```python
from build123d import *

# Parameters (mm, degrees)
EXTRUDE1_DEPTH     = 7.595616
EXTRUDE2_DEPTH     = 3.000375
CIRPATTERN1_COUNT  = 2
CIRPATTERN1_ANGLE  = 90
SKETCH4_R          = 5.969
CUT_EXTRUDE1_DEPTH = 39.496492
SKETCH7_R          = 1.8161
CUT_EXTRUDE2_DEPTH = 70.535078783


with BuildPart() as part:
    # Sketch1 → Revolve1 (revolve)
    with BuildSketch(Plane.XY, mode=Mode.PRIVATE) as revolve1_sk:
        Polygon((34.0487, 5.969), (34.0487, 7.1628), (32.5165085, 7.1628), (21.791168, 9.0424), (21.791168, 7.23392), (8.852662, 7.23392), (8.852662, 9.94664), (5.447792, 9.94664), (5.447792, 7.957312), (-5.447792, 7.957312), (-5.447792, 9.94664), (-8.852662, 9.94664), (-8.852662, 2.8575), (-25.6667, 2.8575), (-25.6667, 3.81), (-33.00095, 2.270125), (-34.0487, 2.270125), (-34.0487, 1.8161), (-5.447792, 1.8161), (-5.447792, 5.969), align=None)
    revolve(revolve1_sk.sketch.rotate(Axis((0, 0, 0), (1, 0, 0)), 90), axis=Axis((0, 0, 0), (1, 0, 0)))

    # Sketch2 → Revolve2 (revolve)
    with BuildSketch(Plane.XY, mode=Mode.PRIVATE) as revolve2_sk:
        with BuildLine():
            Line((10.661142, 7.23392), (8.852662, 7.23392))
            Line((8.852662, 7.23392), (8.852662, 9.0424))
            ThreePointArc((8.852662, 9.0424), (9.382353528, 7.763611528), (10.661142, 7.23392))
        make_face()
        with BuildLine():
            Line((5.447792, 9.94664), (5.447792, 7.957312))
            Line((5.447792, 7.957312), (3.458464, 7.957312))
            ThreePointArc((3.458464, 7.957312), (4.865131319, 8.539972681), (5.447792, 9.94664))
        make_face()
        with BuildLine():
            Line((-5.447792, 9.94664), (-5.447792, 7.957312))
            Line((-5.447792, 7.957312), (-3.458464, 7.957312))
            ThreePointArc((-3.458464, 7.957312), (-4.865131319, 8.539972681), (-5.447792, 9.94664))
        make_face()
        with BuildLine():
            Line((-12.397232, 2.8575), (-8.852662, 2.8575))
            Line((-8.852662, 2.8575), (-8.852662, 6.40207))
            ThreePointArc((-8.852662, 6.40207), (-9.890842517, 3.895680517), (-12.397232, 2.8575))
        make_face()
    revolve(revolve2_sk.sketch.rotate(Axis((0, 0, 0), (1, 0, 0)), 90), axis=Axis((0, 0, 0), (1, 0, 0)))

    # Sketch3 → Extrude1 (add, symmetric)
    with BuildSketch(Plane(origin=(0, 0, 0), x_dir=(-1, 0, 0), z_dir=(0, 0.7071067811865488, 0.7071067811865462))):
        with BuildLine():
            Line((-13.282242083, 0.76609575), (-19.170067917, 0.76609575))
            ThreePointArc((-19.170067917, 0.76609575), (-19.936163667, 0), (-19.170067917, -0.76609575))
            Line((-19.170067917, -0.76609575), (-13.282242083, -0.76609575))
            ThreePointArc((-13.282242083, -0.76609575), (-12.516146333, 0), (-13.282242083, 0.76609575))
        make_face()
    extrude1 = extrude(amount=EXTRUDE1_DEPTH, both=True)

    # Sketch6 → Extrude2 (add, symmetric)
    with BuildSketch(Plane(origin=(0, 0, 0), x_dir=(-1, 0, 0), z_dir=(0, 0.7071067811865488, 0.7071067811865462))):
        with BuildLine():
            Line((15.132685, 0.523875), (22.931247, 0.523875))
            ThreePointArc((22.931247, 0.523875), (23.455122, 0), (22.931247, -0.523875))
            Line((22.931247, -0.523875), (15.132685, -0.523875))
            ThreePointArc((15.132685, -0.523875), (14.60881, 0), (15.132685, 0.523875))
        make_face()
    extrude2 = extrude(amount=EXTRUDE2_DEPTH, both=True)

    # CirPattern1: Extrude1, Extrude2 ×2 about axis
    cirpattern1_axis = Axis((0, 0, 0), (1, 0, 0))
    add([extrude1.rotate(cirpattern1_axis, i * CIRPATTERN1_ANGLE / (CIRPATTERN1_COUNT - 1)) for i in range(1, CIRPATTERN1_COUNT)])
    add([extrude2.rotate(cirpattern1_axis, i * CIRPATTERN1_ANGLE / (CIRPATTERN1_COUNT - 1)) for i in range(1, CIRPATTERN1_COUNT)])

    # Sketch4 → Cut-Extrude1 (cut)
    with BuildSketch(Plane(origin=(34.0487, 0, 0), x_dir=(0, 0, -1), z_dir=(1, 0, 0))):
        with Locations(Location((0, 0, 0), (0, 0, 180))):
            Circle(SKETCH4_R)
    extrude(amount=-CUT_EXTRUDE1_DEPTH, mode=Mode.SUBTRACT)

    # Sketch7 → Cut-Extrude2 (cut, through all)
    with BuildSketch(Plane.ZY.offset(34.0487)):
        Circle(SKETCH7_R)
    extrude(amount=-CUT_EXTRUDE2_DEPTH, mode=Mode.SUBTRACT)


solid = part.part
```
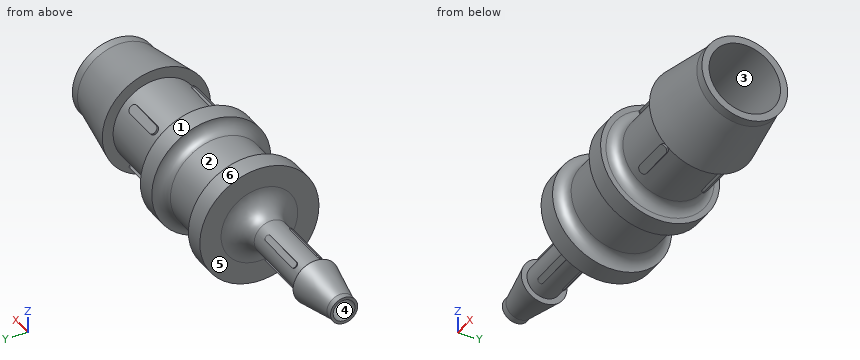
Source: CAD feature listing. Evaluate the final solid. Frame: model axes, mm. Face numbers are marked on the shaded views. A direction names the side the tool comes from. Round coordinates to 2 decimals unless told otherwise and drop trailing zeros. Loops run counter-clockwise (first coordinate to the right, second up) from the corner with the lowest first, then second, coordinate; pieces in that order, holes last. Notation, with made-up numbers: M 63,-3 L 103,-3 A28 cw 103,23 Z; hole C 8,49.5 d6. An arc over 180 degrees is marked long. Use a Markdown table: item, result. Add a question column.
1. Reachability of the marked faces 1, 2 and 3 from +Z, -Z, +X, -X, +Y, -Y: full face, straight path, thin tool, end or side. Return the list, or none.
2. Section query A-A on x = -11.5. Return the cut outline in (y, z).
3. Mould query, pull axis Y, two halves, no side actions, for the marked faces 4, 5 and 6. Classes: pulls with the +Y half, pulls with the -Y half, needs draft (parallel to the pull), parting line crosses it, or undercut.
4. Contact query for flat-ended pins moving along their axis: P1, Ø6, axis at x = 5.5, y = -3.5, coming from the -Z side; P2, Ø3, axis at x = -17.5, z = -2, coming from the -Y side; P3, Ø5, axis at x = 13, y = 2.5, coming from the -Z side. Output: stop coordinate, or through.
5. Line query: line 1 (X direction, y = 5, z = -8.5); line 2 (X direction, y = -4.5, z = 5.5); line 3 (Y direction, x = 11, z = 2.25). Output: solid intervals per line, ascending.
Reported:
| question | item | result |
|---|---|---|
| 1 | face 1 | +X, -X |
| 1 | face 2 | none |
| 1 | face 3 | +X |
| 2 | outline | C 0,0 d5.95; hole C 0,0 d3.63 |
| 3 | face 4 | undercut |
| 3 | face 5 | needs draft |
| 3 | face 6 | parting line crosses it |
| 4 | P1 | stops at z = -9.93 |
| 4 | P2 | stops at y = -2.81 |
| 4 | P3 | stops at z = -7.23 |
| 5 | line 1 | x = -8.85 to -5.45, 5.45 to 8.85 |
| 5 | line 2 | x = -8.85 to 34.05 |
| 5 | line 3 | y = -6.88 to -5.53, 5.53 to 6.88 |
